For this review, take the finished solid that the model builds, in its own axes (mm). Coordinates: 2 decimals unless noted, no trailing zeros. Order: outer loops, then holes, each group sorted by start corner. A loop starts at its lowest first (then second) coordinate and runs counter-clockwise, first axis right, second up. Notation, with made-up numbers: M -23,-30.5 L 12,-30.5 A19 cw 12,-12.5 Z; hole C 25,13 d5. An arc over 180 degrees is marked long. Use one line per item in the form item = value. Start each with the question number.
```python
from build123d import *

# Parameters (mm, degrees)
SKETCH1_W           = 204
SKETCH1_H           = 65
SKETCH1_R           = 2
BOSS_EXTRUDE1_DEPTH = 1.5
FILLET1_R           = 5


with BuildPart() as part:
    # Sketch1 → Boss-Extrude1 (new, symmetric)
    with BuildSketch(Plane.XY):
        Rectangle(SKETCH1_W, SKETCH1_H)
        with Locations((95, -25.5)):
            Circle(SKETCH1_R, mode=Mode.SUBTRACT)
        with Locations((95, 25.5)):
            Circle(SKETCH1_R, mode=Mode.SUBTRACT)
        with Locations((-95, 25.5)):
            Circle(SKETCH1_R, mode=Mode.SUBTRACT)
        with Locations((-95, -25.5)):
            Circle(SKETCH1_R, mode=Mode.SUBTRACT)
    extrude(amount=BOSS_EXTRUDE1_DEPTH, both=True)

    # Fillet1
    fillet1_edges = [part.edges().sort_by_distance(p)[0] for p in [
        (102, -32.5, 0),
        (-102, -32.5, 0),
        (-102, 32.5, 0),
        (102, 32.5, 0),
    ]]
    fillet(fillet1_edges, radius=FILLET1_R)


solid = part.part
```
1. Consider section B-B, the plane y = 25.5. Write out the cut boundary in (x, z).
2. The part is to be moulded in two halves that separate along Y. For faces 1 (the flat face through (-1, 0, -1.5)), 2 (the cylindrical face through (-93.092, 26.101, -0.021)), 3 (the cylindrical face through (96.908, -24.899, -0.021)), 4 (the cylindrical face through (-100.57, 31, -0.02)), say which applies: pulls with the +Y half, pulls with the -Y half, needs draft (parallel to the pull), parting line crosses it, or undercut.
3. For pin 1 Ø3 at (x, y) = (-95, 25.5) entering from +Z; pin 2 Ø5 at (x, y) = (-95, -25.5) entering from -Z, all flat-tipped, find the tip position at first contact; note any pin that passes through.
4. To check wall thickness, follow line 1 (Y direction, x = 95, z = 0); line 2 (X direction, y = -26, z = -0.65); line 3 (X direction, y = 24.5, z = 0.95). State the ranges of each line that lie inside material, in increasing order.
5. Consider section A-A, the plane x = 95. Write out the cut boundary in (y, z).
Answers follow:
q1.outline = M -102,-1.5 L -97,-1.5 L -97,1.5 L -102,1.5 Z; M -93,-1.5 L 93,-1.5 L 93,1.5 L -93,1.5 Z; M 97,-1.5 L 102,-1.5 L 102,1.5 L 97,1.5 Z
q2.face_1 = needs draft
q2.face_2 = undercut
q2.face_3 = undercut
q2.face_4 = pulls with the +Y half
q3.pin_1 = through
q3.pin_2 = -1.5
q4.line_1 = -32.5 to -27.5, -23.5 to 23.5, 27.5 to 32.5
q4.line_2 = -102 to -96.94, -93.06 to 93.06, 96.94 to 102
q4.line_3 = -102 to -96.73, -93.27 to 93.27, 96.73 to 102
q5.outline = M -32.5,-1.5 L -27.5,-1.5 L -27.5,1.5 L -32.5,1.5 Z; M -23.5,-1.5 L 23.5,-1.5 L 23.5,1.5 L -23.5,1.5 Z; M 27.5,-1.5 L 32.5,-1.5 L 32.5,1.5 L 27.5,1.5 Z
